Read the model definition and answer for the solid it produces. Units are mm, in the model's axes. A direction names the side the tool comes from. Coordinates: 2 decimals unless noted, no trailing zeros. Write each loop counter-clockwise with the first axis right and the second up, starting at its lowest first coordinate (ties: lowest second). Pieces come first, ordered by that corner, then holes. Notation, with made-up numbers: (-1.5, 67) -> (55.5, 67) arc R29 ccw to (55.5, 104) -> close; hole circle Ø10 at (11.5, 86.5). An arc over 180 degrees is marked (long way). Write item = value, one per line. Start each with the question number.
1) A tool of negligible diameter and unlimited length cuts with its end or side. For faces 3 (the face through (789.22, -119.68, 3.13)), 4 (the face through (426, -433, 0)), from which of +Z, -Z, +X, -X, +Y, -Y can it reach the whole face along a straight path? Write none if from no direction.
2) Section D-D (z = 1.5) is taken. Count the separate pieces of the cut face and the enclosed holes in it, plus the area to 3 significant figures.
3) Section C-C (x = 695) is taken. Determine the outline of the cut face in (y, z), plus the area to 3 significant figures.
4) Section B-B (y = -91) is taken. Determine the outline of the cut face in (x, z).
5) Section A-A (x = 531) is taken. Determine the outline of the cut face in (y, z).
6) For a pull along Y with two mould halves and no side action, classify faces 1 (the face through (426, -433, 6.35)), 2 (the face through (358.04, -494.43, 3.22)) as released by +Y, released by -Y, zero draft, split by the parting line, or undercut.
7) Find the intervals of material crossed by line 1 along Y through (x, z) = (695, 5.5); line 2 along Y through (x, z) = (444, 0.75); line 3 along Y through (x, z) = (434.5, 3), in increasing order. Write a range as from..to.
from build123d import *

# Parameters (mm, degrees)
SKETCH1_W           = 874.1918
SKETCH1_H           = 712.1144
BOSS_EXTRUDE1_DEPTH = 6.35
SKETCH2_R           = 53.975
CUT_EXTRUDE1_DEPTH  = 1126.241709767
SKETCH3_R           = 3.81
CUT_EXTRUDE2_DEPTH  = 1126.241709767
SKETCH4_R           = 13.97
CUT_EXTRUDE3_DEPTH  = 1126.241709767
SKETCH5_W           = 99.06
SKETCH5_H           = 50.8
CUT_EXTRUDE4_DEPTH  = 1126.241709767
SKETCH6_R           = 3.175
CUT_EXTRUDE5_DEPTH  = 1126.241709767
CUT_EXTRUDE7_DEPTH  = 1126.241709767
SKETCH9_W           = 144.78
SKETCH9_H           = 53.34
CUT_EXTRUDE8_DEPTH  = 1126.241709767
SKETCH10_W          = 557.53
SKETCH10_H          = 363.982
CUT_EXTRUDE9_DEPTH  = 1126.241709767
SKETCH12_R          = 2.54
CUT_EXTRUDE11_DEPTH = 1126.241709767


with BuildPart() as part:
    # Sketch1 → Boss-Extrude1 (new body)
    with BuildSketch(Plane.XY):
        with Locations((431.8, -358.8893)):
            Rectangle(SKETCH1_W, SKETCH1_H)
    extrude(amount=BOSS_EXTRUDE1_DEPTH)

    # Sketch2 → Cut-Extrude1 (cut, through all)
    with BuildSketch(Plane.XY.offset(6.35)):
        with Locations((165.1381, -448.3735)):
            Circle(SKETCH2_R)
        with Locations((698.5381, -448.3735)):
            Circle(SKETCH2_R)
        with Locations((698.5381, -596.4555)):
            Circle(SKETCH2_R)
    extrude(amount=-CUT_EXTRUDE1_DEPTH, mode=Mode.SUBTRACT)

    # Sketch3 → Cut-Extrude2 (cut, through all)
    with BuildSketch(Plane.XY.offset(6.35)):
        with Locations((122.0851, -405.3205)):
            Circle(SKETCH3_R)
        with Locations((208.1911, -491.4265)):
            Circle(SKETCH3_R)
        with Locations((122.0851, -491.4265)):
            Circle(SKETCH3_R)
        with Locations((741.5911, -405.3205)):
            Circle(SKETCH3_R)
        with Locations((655.4851, -405.3205)):
            Circle(SKETCH3_R)
        with Locations((655.4851, -491.4265)):
            Circle(SKETCH3_R)
        with Locations((741.5911, -491.4265)):
            Circle(SKETCH3_R)
        with Locations((741.5911, -553.4025)):
            Circle(SKETCH3_R)
        with Locations((655.4851, -553.4025)):
            Circle(SKETCH3_R)
        with Locations((655.4851, -639.5085)):
            Circle(SKETCH3_R)
        with Locations((741.5911, -639.5085)):
            Circle(SKETCH3_R)
        with Locations((208.1911, -405.3205)):
            Circle(SKETCH3_R)
    extrude(amount=-CUT_EXTRUDE2_DEPTH, mode=Mode.SUBTRACT)

    # Sketch4 → Cut-Extrude3 (cut, through all)
    with BuildSketch(Plane.XY.offset(6.35)):
        with Locations((368.3381, -427.6725)):
            Circle(SKETCH4_R)
        with Locations((368.3381, -465.7725)):
            Circle(SKETCH4_R)
        with Locations((368.3381, -503.8725)):
            Circle(SKETCH4_R)
        with Locations((368.3381, -541.9725)):
            Circle(SKETCH4_R)
    extrude(amount=-CUT_EXTRUDE3_DEPTH, mode=Mode.SUBTRACT)

    # Sketch5 → Cut-Extrude4 (cut, through all)
    with BuildSketch(Plane.XY.offset(6.35)):
        with Locations((431.8381, -622.2365)):
            Rectangle(SKETCH5_W, SKETCH5_H)
    extrude(amount=-CUT_EXTRUDE4_DEPTH, mode=Mode.SUBTRACT)

    # Sketch6 → Cut-Extrude5 (cut, through all)
    with BuildSketch(Plane.XY.offset(6.35)):
        with Locations((131.6101, -522.4145)):
            Circle(SKETCH6_R)
        with Locations((198.6661, -522.4145)):
            Circle(SKETCH6_R)
        with Locations((131.6101, -670.4965)):
            Circle(SKETCH6_R)
        with Locations((198.6661, -670.4965)):
            Circle(SKETCH6_R)
        with Locations((398.3101, -670.4965)):
            Circle(SKETCH6_R)
        with Locations((465.3661, -670.4965)):
            Circle(SKETCH6_R)
        with Locations((419.9001, -427.9265)):
            Circle(SKETCH6_R)
        with Locations((486.9561, -427.9265)):
            Circle(SKETCH6_R)
        with Locations((419.9001, -466.0265)):
            Circle(SKETCH6_R)
        with Locations((486.9561, -466.0265)):
            Circle(SKETCH6_R)
        with Locations((419.9001, -504.1265)):
            Circle(SKETCH6_R)
        with Locations((486.9561, -504.1265)):
            Circle(SKETCH6_R)
        with Locations((419.9001, -542.2265)):
            Circle(SKETCH6_R)
        with Locations((486.9561, -542.2265)):
            Circle(SKETCH6_R)
        with Locations((665.0101, -522.4145)):
            Circle(SKETCH6_R)
        with Locations((732.0661, -522.4145)):
            Circle(SKETCH6_R)
        with Locations((665.0101, -670.4965)):
            Circle(SKETCH6_R)
        with Locations((732.0661, -670.4965)):
            Circle(SKETCH6_R)
    extrude(amount=-CUT_EXTRUDE5_DEPTH, mode=Mode.SUBTRACT)

    # Sketch8 → Cut-Extrude7 (cut, through all)
    with BuildSketch(Plane(origin=(0, 0, 0), x_dir=(-1, 0, 0), z_dir=(0, 0, -1))):
        with BuildLine():
            Line((-109.32724398, -145.8341), (-114.0206, -145.8341))
            Line((-114.0206, -145.8341), (-114.0206, -164.6301))
            Line((-114.0206, -164.6301), (-109.32724398, -164.6301))
            ThreePointArc((-109.32724398, -164.6301), (-75.0316, -190.7921), (-40.73595602, -164.6301))
            Line((-40.73595602, -164.6301), (-36.0426, -164.6301))
            Line((-36.0426, -164.6301), (-36.0426, -145.8341))
            Line((-36.0426, -145.8341), (-40.73595602, -145.8341))
            ThreePointArc((-40.73595602, -145.8341), (-75.0316, -119.6721), (-109.32724398, -145.8341))
        make_face()
        with BuildLine():
            Line((-749.5794, -164.6301), (-754.27275602, -164.6301))
            ThreePointArc((-754.27275602, -164.6301), (-788.5684, -190.7921), (-822.86404398, -164.6301))
            Line((-822.86404398, -164.6301), (-827.5574, -164.6301))
            Line((-827.5574, -164.6301), (-827.5574, -145.8341))
            Line((-827.5574, -145.8341), (-822.86404398, -145.8341))
            ThreePointArc((-822.86404398, -145.8341), (-788.5684, -119.6721), (-754.27275602, -145.8341))
            Line((-754.27275602, -145.8341), (-749.5794, -145.8341))
            Line((-749.5794, -145.8341), (-749.5794, -164.6301))
        make_face()
    extrude(amount=-CUT_EXTRUDE7_DEPTH, mode=Mode.SUBTRACT)

    # Sketch9 → Cut-Extrude8 (cut, through all)
    with BuildSketch(Plane.XY.offset(6.35)):
        with Locations((162.5981, -613.3465)):
            Rectangle(SKETCH9_W, SKETCH9_H)
    extrude(amount=-CUT_EXTRUDE8_DEPTH, mode=Mode.SUBTRACT)

    # Sketch10 → Cut-Extrude9 (cut, through all)
    with BuildSketch(Plane.XY.offset(6.35)):
        with Locations((436.0291, -205.946512668)):
            Rectangle(SKETCH10_W, SKETCH10_H)
    extrude(amount=-CUT_EXTRUDE9_DEPTH, mode=Mode.SUBTRACT)

    # Sketch12 → Cut-Extrude11 (cut, through all)
    with BuildSketch(Plane(origin=(0, 0, 0), x_dir=(-1, 0, 0), z_dir=(0, 0, -1))):
        with Locations((-444.5381, -587.9465)):
            Circle(SKETCH12_R)
        with Locations((-419.1381, -587.9465)):
            Circle(SKETCH12_R)
    extrude(amount=-CUT_EXTRUDE11_DEPTH, mode=Mode.SUBTRACT)


solid = part.part
Answer key:
q1.face_3 = +Z, -Z
q1.face_4 = -Z, +X, -X, +Y, -Y
q2.separate_pieces = 1
q2.enclosed_holes = 44
q2.area = 368,000 mm^2
q3.outline = (-714.95, 0) -> (-650.31, 0) -> (-650.31, 6.35) -> (-714.95, 6.35) -> close; (-542.6, 0) -> (-502.23, 0) -> (-502.23, 6.35) -> (-542.6, 6.35) -> close; (-394.51, 0) -> (-387.94, 0) -> (-387.94, 6.35) -> (-394.51, 6.35) -> close; (-23.96, 0) -> (-2.83, 0) -> (-2.83, 6.35) -> (-23.96, 6.35) -> close
q3.area = 843 mm^2
q4.outline = (-5.3, 0) -> (157.26, 0) -> (157.26, 6.35) -> (-5.3, 6.35) -> close; (714.79, 0) -> (868.9, 0) -> (868.9, 6.35) -> (714.79, 6.35) -> close
q5.outline = (-714.95, 0) -> (-387.94, 0) -> (-387.94, 6.35) -> (-714.95, 6.35) -> close; (-23.96, 0) -> (-2.83, 0) -> (-2.83, 6.35) -> (-23.96, 6.35) -> close
q6.face_1 = zero draft
q6.face_2 = undercut
q7.line_1 = -714.95..-650.31, -542.6..-502.23, -394.51..-387.94, -23.96..-2.83
q7.line_2 = -714.95..-647.64, -596.84..-590.43, -585.46..-387.94, -23.96..-2.83
q7.line_3 = -714.95..-647.64, -596.84..-387.94, -23.96..-2.83
